Input: part model. Units: mm. Frame: model coordinates. A direction names the side the tool comes from. Round coordinates to 2 decimals unless told otherwise and drop trailing zeros. Loops run counter-clockwise (first coordinate to the right, second up) from the corner with the lowest first, then second, coordinate; pieces in that order, holes last.
(1) Cut plane B-B, the plane x = -135. Output: boundary loops of the cut face in (y, z).
(2) First-contact query: pin 1 Ø12 at (y, z) = (75, -346.5) entering from -X; pin 2 Ø8 at (y, z) = (19.5, -109.5) entering from -X; pin 3 Ø4 at (x, z) = (92, -329) entering from +Y. Flat tips, straight axial feed; report the tip coordinate or a pass-through.
(3) Line query: line 1 (Y direction, x = -4.5, z = 0); line 2 (Y direction, x = -13.5, z = -278.5); line 3 (X direction, y = 103.5, z = -343). Output: solid intervals per line, ascending.
(4) Access query for faces 1 (the face through (-112.5, -49, -1)), 2 (the face through (1.505, 114.374, -85.649)), 3 (the face through (109.965, 66.538, 34.608)), 4 (the face through (-107.743, 12.839, 40.769)), 5 (the face through (107.5, 196, -271)). Directions: +Z, -Z, +X, -X, +Y, -Y. A direction counts if a zero-diameter tool reaches every point of the face in a straight line with its end or side. Return the directions, or none.
(5) Cut plane A-A, the plane x = -10.5. Output: boundary loops of the cut face in (y, z), and give its area (3 significant figures).
(6) Draft query along Z for faces 6 (the face through (1.505, 880.744, -319.651)), 7 (the face through (112.5, 49, -1)), 8 (the face through (-110.035, 74.362, -9.764)). Return one class per face: released by +Z, released by -Z, zero draft, split by the parting line, or undercut.
from build123d import *

# Parameters (mm, degrees)
SKETCH1_R           = 42.5
BOSS_EXTRUDE1_DEPTH = 107.5
SKETCH2_R           = 75
SKETCH2_R_2         = 42.5
BOSS_EXTRUDE2_DEPTH = 5
BOSS_EXTRUDE3_START = 5
SKETCH3_R           = 75
SKETCH3_R_2         = 42.5
BOSS_EXTRUDE3_DEPTH = 5
CHAMFER1_SIZE       = 5
BOSS_EXTRUDE4_DEPTH = 75
BOSS_EXTRUDE5_START = 75
BOSS_EXTRUDE5_DEPTH = 75
FILLET2_R           = 15
SKETCH7_R           = 42.5
BOSS_EXTRUDE6_DEPTH = 215


with BuildPart() as part:
    # Sketch1 → Boss-Extrude1 (new, symmetric)
    with BuildSketch(Plane(origin=(0, 0, 0), x_dir=(0, 0, -1), z_dir=(1, 0, 0))):
        with BuildLine():
            ThreePointArc((-4.759905033, 92.377450193), (-85.458856757, -35.398217494), (61.954960333, -68.686482587))
            ThreePointArc((61.954960333, -68.686482587), (140.229582164, -20.76943431), (230.521573397, -4.328136996))
            ThreePointArc((230.521573397, -4.328136996), (323.357836379, 133.939201328), (159.94291274, 166.063822779))
            ThreePointArc((159.94291274, 166.063822779), (84.471080629, 113.843496313), (-4.759905033, 92.377450193))
        make_face()
        Circle(SKETCH1_R, mode=Mode.SUBTRACT)
    extrude(amount=BOSS_EXTRUDE1_DEPTH, both=True)

    # Sketch2 → Boss-Extrude2 (add)
    with BuildSketch(Plane(origin=(107.5, 0, 0), x_dir=(0, 0, -1), z_dir=(1, 0, 0))):
        with Locations(Location((0, 0, 0), (0, 0, 180))):
            Circle(SKETCH2_R)
        Circle(SKETCH2_R_2, mode=Mode.SUBTRACT)
    extrude(amount=BOSS_EXTRUDE2_DEPTH)

    # Sketch3 → Boss-Extrude3 (add)
    with BuildSketch(Plane.ZY.offset(107.5).offset(BOSS_EXTRUDE3_START)):
        Circle(SKETCH3_R)
        Circle(SKETCH3_R_2, mode=Mode.SUBTRACT)
    extrude(amount=-BOSS_EXTRUDE3_DEPTH)

    # Chamfer1
    # the kernel refuses this chamfer: 5 mm, written as the material it takes off along each edge
    with BuildSketch(Plane(origin=(112.5, 0, 0), x_dir=(0, 0, -1), z_dir=(0, -1, 0))) as chamfer1_piece_1:
        Polygon((42.5 + CHAMFER1_SIZE, 0), (42.5, -CHAMFER1_SIZE), (42.5, 0), align=None)
    revolve(axis=Axis((112.5, 0, 0), (1, 0, 0)), mode=Mode.SUBTRACT)
    with BuildSketch(Plane(origin=(-112.5, 0, 0), x_dir=(0, 0, 1), z_dir=(0, -1, 0))) as chamfer1_piece_2:
        Polygon((42.5 + CHAMFER1_SIZE, 0), (42.5, -CHAMFER1_SIZE), (42.5, 0), align=None)
    revolve(axis=Axis((-112.5, 0, 0), (-1, 0, 0)), mode=Mode.SUBTRACT)

    # Sketch5 → Boss-Extrude4 (add)
    with BuildSketch(Plane.ZY.offset(107.5)):
        with BuildLine():
            ThreePointArc((-335.722160279, 54.643910463), (-186.43026552, -7.636801177), (-129.224593262, 143.672378798))
            ThreePointArc((-129.224593262, 143.672378798), (-232.809942482, 478.212645548), (-239.526554212, 828.358332052))
            ThreePointArc((-239.526554212, 828.358332052), (-315.830208714, 928.305649758), (-417.57768021, 854.419480204))
            ThreePointArc((-417.57768021, 854.419480204), (-431.229967878, 448.945530482), (-335.722160279, 54.643910463))
        make_face()
    extrude(amount=BOSS_EXTRUDE4_DEPTH)

    # Sketch6 → Boss-Extrude5 (add)
    with BuildSketch(Plane(origin=(107.5, 0, 0), x_dir=(0, 0, -1), z_dir=(1, 0, 0)).offset(BOSS_EXTRUDE5_START)):
        with BuildLine():
            ThreePointArc((129.224593262, 143.672378798), (232.809942482, 478.212645548), (239.526554212, 828.358332052))
            ThreePointArc((239.526554212, 828.358332052), (315.830208714, 928.305649758), (417.57768021, 854.419480204))
            ThreePointArc((417.57768021, 854.419480204), (431.229967878, 448.945530482), (335.722160279, 54.643910463))
            ThreePointArc((335.722160279, 54.643910463), (186.43026552, -7.636801177), (129.224593262, 143.672378798))
        make_face()
    extrude(amount=-BOSS_EXTRUDE5_DEPTH)

    # Fillet2
    fillet2_edges = [part.edges().sort_by_distance(p)[0] for p in [
        (-182.5, 478.212645548, -232.809942482),
        (-182.5, 928.305649758, -315.830208714),
        (-182.5, 448.945530482, -431.229967878),
        (-182.5, -7.636801177, -186.43026552),
        (182.5, -7.636801177, -186.43026552),
        (182.5, 448.945530482, -431.229967878),
        (182.5, 928.305649758, -315.830208714),
        (182.5, 478.212645548, -232.809942482),
    ]]
    fillet(fillet2_edges, radius=FILLET2_R)

    # Sketch7 → Boss-Extrude6 (add)
    with BuildSketch(Plane.ZY.offset(-107.5)):
        with Locations(Location((-328.864527293, 839.254504122, 0), (0, 0, 180))):
            Circle(SKETCH7_R)
        with BuildLine():
            ThreePointArc((-430.016772116, 765.815935458), (-433.115150694, 468.647268594), (-377.566301605, 176.700112622))
            ThreePointArc((-377.566301605, 176.700112622), (-290.266675416, 252.323787921), (-174.772654288, 253.462244012))
            ThreePointArc((-174.772654288, 253.462244012), (-235.480184212, 495.562856506), (-246.877162179, 744.898412841))
            ThreePointArc((-246.877162179, 744.898412841), (-343.049337537, 715.061947347), (-430.016772116, 765.815935458))
        make_face()
    extrude(amount=BOSS_EXTRUDE6_DEPTH)


solid = part.part
Reported:
1. outline: (54.64, -335.72) arc R1500 ccw to (854.42, -417.58) arc R90 ccw to (828.36, -239.53) arc R1250 cw to (143.67, -129.22) arc R112.5 ccw (long way) to start
2. pin 1: stops at x = -176.78
2. pin 2: stops at x = -107.5
2. pin 3: stops at y = 881.75
3. line 1: y = -92.5 to -42.5, 42.5 to 92.67
3. line 2: y = 7.69 to 183.65, 256.29 to 724.85
3. line 3: x = -181.73 to -107.5, 107.5 to 181.73
4. face 1: +Z, -X, +Y, -Y
4. face 2: +Z, +Y
4. face 3: +X
4. face 4: -X
4. face 5: none
5. outline: (-68.69, -61.95) arc R250 cw to (-4.33, -230.52) arc R100 ccw (long way) to (166.06, -159.94) arc R250 cw to (92.38, 4.76) arc R92.5 ccw (long way) to start; (176.7, -377.57) arc R1500 ccw to (765.82, -430.02) arc R125 cw to (744.9, -246.88) arc R1250 cw to (253.46, -174.77) arc R167.5 cw to start; circle Ø85 at (839.25, -328.86); hole circle Ø85 at (0, 0)
5. area: 169,000 mm2
6. face 6: split by the parting line
6. face 7: zero draft
6. face 8: undercut
